For this review, use the dimensioned drawing (mm, ordinates from the lowest corner) and the shaded views. A direction names the side the tool comes from. Give positions to 0.01 mm unless a question says otherwise; leave off trailing zeros. Write each loop counter-clockwise with the first axis right and the second up, starting at its lowest first coordinate (ties: lowest second). Pieces come first, ordered by that corner, then holes. Notation, with made-up numbers: (26.25, -31.5) -> (31.25, -31.5) arc R9 cw to (31.25, -14.5) -> close; hole circle Ø10 at (-4, -24.75). An arc over 180 degrees is marked (long way). Answer as CSV lines item,"result".
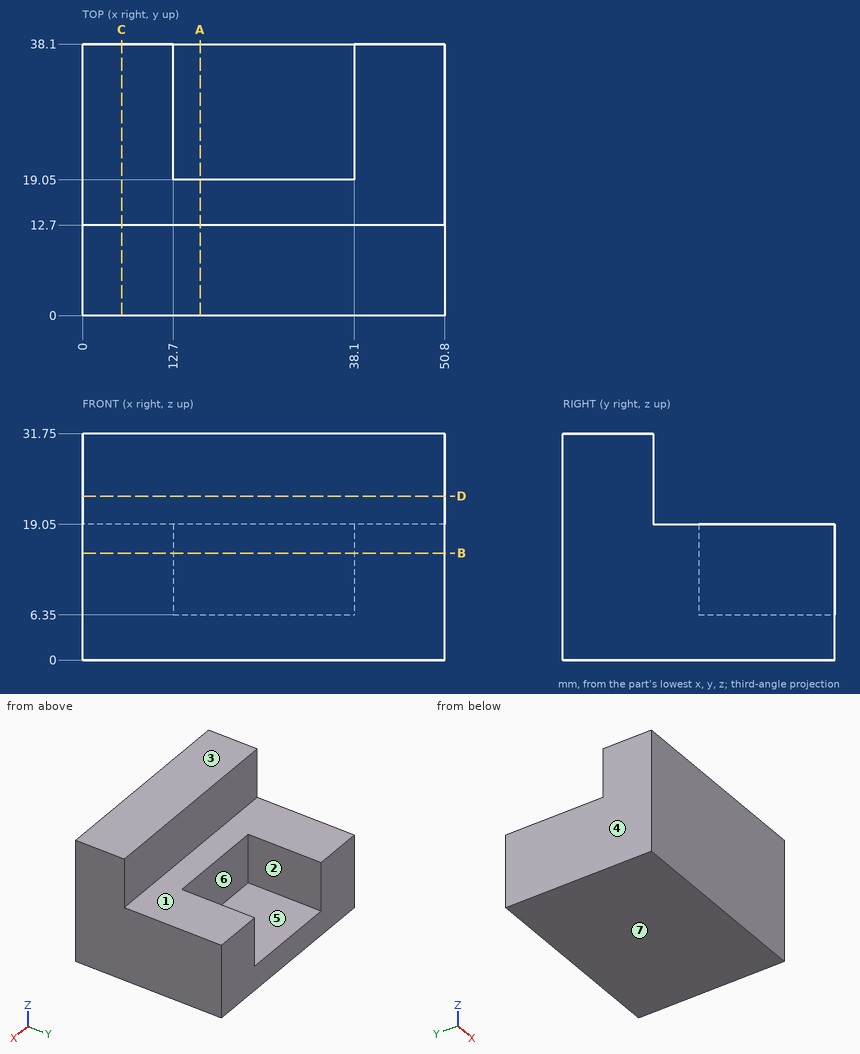
Q1. Add section A-A (x = 16.5). Write out the cut boundary in (y, z).
Answer block:
outline,"(0, 0) -> (38.1, 0) -> (38.1, 6.35) -> (19.05, 6.35) -> (19.05, 19.05) -> (12.7, 19.05) -> (12.7, 31.75) -> (0, 31.75) -> close"
Q2. Add section B-B (z = 15). Write out the cut boundary in (x, y).
Answer block:
outline,"(0, 0) -> (50.8, 0) -> (50.8, 38.1) -> (38.1, 38.1) -> (38.1, 19.05) -> (12.7, 19.05) -> (12.7, 38.1) -> (0, 38.1) -> close"
Q3. Add section C-C (x = 5.5). Write out the cut boundary in (y, z).
Answer block:
outline,"(0, 0) -> (38.1, 0) -> (38.1, 19.05) -> (12.7, 19.05) -> (12.7, 31.75) -> (0, 31.75) -> close"
Q4. To check wall thickness, follow probe 1 along X at (y, z) = (27, 9.5); probe 2 along Y at (x, z) = (34, 26); probe 3 along Y at (x, z) = (23.5, 15.5). State the ranges of each line that lie inside material, in increasing order. Write a range as [from, to].
Answer block:
probe 1,"x = [0, 12.7], [38.1, 50.8]"
probe 2,"y = [0, 12.7]"
probe 3,"y = [0, 19.05]"
Q5. For the marked faces 1, 2 and 3, list the 3-axis set-ups (+Z, -Z, +X, -X, +Y, -Y) from which the entire face can be reached by the end or side of a thin tool; tool diameter is ignored.
Answer block:
face 1,"+Z, +X, -X, +Y"
face 2,"+Z, +Y"
face 3,"+Z, +X, -X, +Y, -Y"
Q6. Add section D-D (z = 23). Write out the cut boundary in (x, y).
Answer block:
outline,"(0, 0) -> (50.8, 0) -> (50.8, 12.7) -> (0, 12.7) -> close"
Q7. Clearance check with flat-ended pins moving along their axes: pin 1 (4 mm diameter, centred on x = 42.5, y = 32.5, fed in from -Z); pin 2 (1.5 mm diameter, centred on x = 29.5, y = 14, fed in from +Z); pin 3 (1.5 mm diameter, centred on x = 20, z = 18.5, fed in from +Y); pin 4 (9.5 mm diameter, centred on x = 23, y = 24, fed in from +Z). State where each tip first meets the part, or that it passes through.
Answer block:
pin 1,"stops at z = 0"
pin 2,"stops at z = 19.05"
pin 3,"stops at y = 19.05"
pin 4,"stops at z = 6.35"
Q8. Draft analysis for pull direction X (two halves, no side actions). For the marked faces 4, 5, 6 and 7, state which applies: released by +X, released by -X, zero draft, split by the parting line, or undercut.
Answer block:
face 4,"released by -X"
face 5,"undercut"
face 6,"undercut"
face 7,"zero draft"
